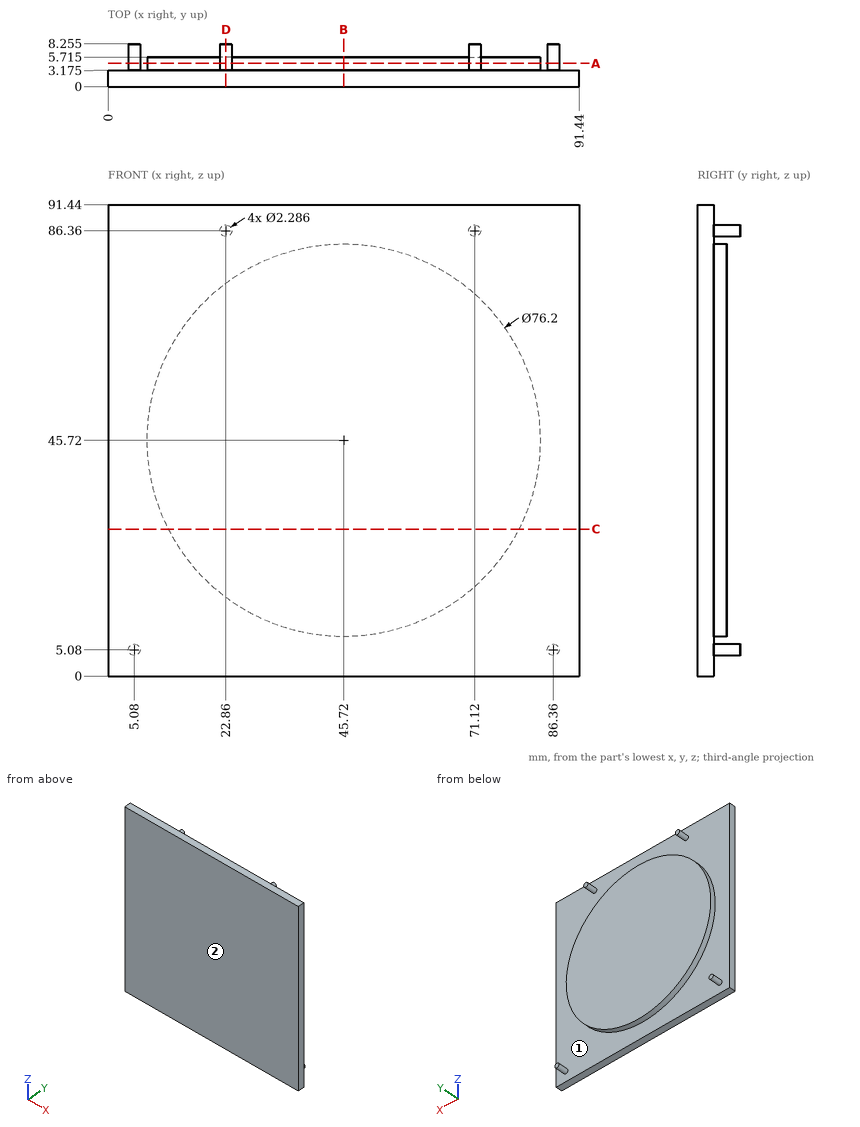
Print and shaded views of the part. All mm, measured from the part's lowest x, y and z. A direction names the side the tool comes from. Give positions to 0.01 mm unless a question says otherwise; leave off trailing zeros. Write each loop counter-clockwise with the first axis right and the second up, starting at its lowest first coordinate (ties: lowest second). Pieces come first, ordered by that corner, then holes. Notation, with made-up numbers: M 26,81.25 L 48,81.25 A29 ccw 48,117.25 Z; hole C -7,4.5 d1. An arc over 180 degrees is marked long. Use a Markdown table: item, result.
1) Drill centre lines: line 1 (Y direction, x = 39.5, z = 73) (3 decimals); line 2 (Y direction, x = 87.5, z = 33.5) (3 decimals); line 3 (X direction, y = 4.5, z = 45). Where is each one in solid material? Low to high. Write a range as from..to.
Responses:
| item | result |
|---|---|
| line 1 | y = 0..5.715 |
| line 2 | y = 0..3.175 |
| line 3 | x = 7.63..83.81 |
2) Tool access for the marked faces 1 and 2: list every direction of +Z, -Z, +X, -X, +Y, -Y with a clear straight run to the whole face (end or side of a thin tool).
Responses:
| item | result |
|---|---|
| face 1 | +Y |
| face 2 | +Z, -Z, +X, -X, -Y |
3) Cut at B-B (x = 45.72). List the corners of the cut face in (y, z) (3 decimals), and give its area (3 significant figures).
Responses:
| item | result |
|---|---|
| outline | M 0,0 L 3.175,0 L 3.175,7.62 L 5.715,7.62 L 5.715,83.82 L 3.175,83.82 L 3.175,91.44 L 0,91.44 Z |
| area | 484 mm2 |
4) Cut at C-C (z = 28.5). List the corners of the cut face in (x, y) (1 decimal).
Responses:
| item | result |
|---|---|
| outline | M 0,0 L 91.4,0 L 91.4,3.2 L 79.7,3.2 L 79.7,5.7 L 11.7,5.7 L 11.7,3.2 L 0,3.2 Z |
5) Cut at A-A (y = 4.5). List the corners of the cut face in (x, z), and give its area (3 significant figures).
Responses:
| item | result |
|---|---|
| outline | C 5.08,5.08 d2.29; C 45.72,45.72 d76.2; C 22.86,86.36 d2.29; C 71.12,86.36 d2.29; C 86.36,5.08 d2.29 |
| area | 4,580 mm2 |
6) Pin check, flat tip, straight feed: pin 1 (3 mm diameter, centred on x = 63.5, y = 6, fed in from +Z). Stop position of the tip, or through.
Responses:
| item | result |
|---|---|
| pin 1 | stops at z = 80.15 |
7) Cut at D-D (x = 22.86). List the corners of the cut face in (y, z) (3 decimals), and give its area (3 significant figures).
Responses:
| item | result |
|---|---|
| outline | M 0,0 L 3.175,0 L 3.175,15.24 L 5.715,15.24 L 5.715,76.2 L 3.175,76.2 L 3.175,85.217 L 8.255,85.217 L 8.255,87.503 L 3.175,87.503 L 3.175,91.44 L 0,91.44 Z |
| area | 457 mm2 |
